Read the model definition and answer for the solid it produces. Units are mm, in the model's axes. A direction names the side the tool comes from. Coordinates: 2 decimals unless noted, no trailing zeros. Write each loop counter-clockwise with the first axis right and the second up, starting at its lowest first coordinate (ties: lowest second). Pieces come first, ordered by that corner, then holes. Notation, with made-up numbers: (51, 66) - (74, 66) arc R12 cw to (74, 74) - close; hole circle Ø10 at (40, -28.5). An arc over 180 degrees is marked (long way). Use a Markdown table: item, result.
Autodesk Inventor part; units mm, degrees
ref_plane "YZ Plane" through (0, 0, 0) normal (1, 0, 0) x (0, 1, 0)
ref_plane "XZ Plane" through (0, 0, 0) normal (0, 1, 0) x (-1, 0, 0)
ref_plane "XY Plane" through (0, 0, 0) normal (0, 0, 1) x (1, 0, 0)
sketch "Sketch1" plane through (0, 0, 0) normal (0, 1, 0) x (-1, 0, 0)
  line L0 (0, 0) -> (70, 0)
  line L1 (70, 0) -> (70, -10)
  line L2 (70, -10) -> (0, -10)
  line L3 (0, -10) -> (0, 0)
  line L4 (70, 0) -> (0, 0)
  line L5 (0, 0) -> (0, -5)
  line L6 (0, -5) -> (70, -5)
  line L7 (70, -5) -> (70, 0)
  line L8 (70, -5) -> (62, -5)
  line L9 (62, -5) -> (44, -5)
  line L10 (44, -5) -> (26, -5)
  line L11 (26, -5) -> (8, -5)
  line L12 (8, -5) -> (-6, -5)
  line L13 (70, 0) -> (90, 0)
  line L14 (90, 0) -> (90, -10)
  line L15 (90, -10) -> (70, -10)
  line L16 (70, -10) -> (70, 0)
  line L17 (0, -10) -> (-22, -10)
  line L18 (-22, -10) -> (-22, 0)
  line L19 (-22, 0) -> (0, 0)
  line L20 (0, 0) -> (0, -10)
  dimension "d0" = 70
  dimension "d1" = 10
  dimension "d2" = 5
  dimension "d3" = 8
  dimension "d4" = 18
  dimension "d5" = 18
  dimension "d6" = 18
  dimension "d22" = 20
  dimension "d23" = 22
extrude "Extrusion1" add sketch "Sketch1" along normal blind 40 contours L0 L1 L6 L3 | L6 L1 L2 L3
hole "Hole1" at (6, 0, -5) at (-8, 0, -5) at (-26, 0, -5) at (-44, 0, -5) at (-62, 0, -5) direction (0, 1, 0) diameter 3.242 depth 15 tip angle 118
extrude "Extrusion3" add sketch "Sketch1" along normal blind 86 contours L3 L17 L18 L19 | L13 L14 L15 L1
sketch "Sketch4" plane through (22, 0, -10) normal (0, 0, -1) x (-1, 0, 0)
  line L0 (112, 0) -> (112, 86)
  line L1 (112, 86) -> (101.5, 86)
  line L2 (101.5, 86) -> (101.5, 76)
  line L3 (101.5, 76) -> (112, 76)
  line L4 (112, 76) -> (112, 86)
  line L5 (0, 86) -> (22, 86)
  line L6 (0, 86) -> (8.5, 86)
  line L7 (8.5, 86) -> (8.5, 76)
  line L8 (8.5, 76) -> (0, 76)
  line L9 (0, 76) -> (0, 86)
  line L10 (22, 40) -> (92, 40)
  line L11 (22, 40) -> (55, 40)
  line L12 (55, 40) -> (55, 29.5)
  line L13 (55, 29.5) -> (22, 29.5)
  line L14 (22, 29.5) -> (22, 40)
  point P0 (22, 0)
  dimension "d35" = 10.5
  dimension "d36" = 10
  dimension "d44" = 8.5
  dimension "d45" = 10
  dimension "d46" = 10.5
  dimension "d47" = 33
hole "Hole3" at (-79.5, 76, -10) at (13.5, 76, -10) at (-33, 29.5, -10) direction (0, 0, 1) diameter 5.2 end through all counterbore diameter 10 counterbore depth 5
properties part number "CameraAdapter_part2"
(1) A cutting plane is placed at B-B, the plane y = 76. Write down the section's boundary in (x, z), and give its area (3 significant figures).
Report:
| item | result |
|---|---|
| outline | (-90, -10) - (-84.5, -10) - (-84.5, -5) - (-82.1, -5) - (-82.1, 0) - (-90, 0) - close; (-76.9, -5) - (-74.5, -5) - (-74.5, -10) - (-70, -10) - (-70, 0) - (-76.9, 0) - close; (0, -10) - (8.5, -10) - (8.5, -5) - (10.9, -5) - (10.9, 0) - (0, 0) - close; (16.1, -5) - (18.5, -5) - (18.5, -10) - (22, -10) - (22, 0) - (16.1, 0) - close |
| area | 268 mm² |
(2) For faces 4 (the flat face through (0, 63, -5)), 5 (the flat face through (-80, 86, -5)), 6 (the cylindrical face through (-45.607, 7.605, -4.789)), 7 (the cylindrical face through (-34.757, 27.584, -2.465)), 8 (the flat face through (16, 78, -5)), determine the directions among +Z, -Z, +X, -X, +Y, -Y from which every point of the face is accessible in a straight line to the end or side of a thin tool.
Report:
| item | result |
|---|---|
| face 4 | +Z, -Z, +Y |
| face 5 | +Z, -Z, +X, -X, +Y |
| face 6 | -Y |
| face 7 | +Z, -Z |
| face 8 | -Z |
(3) A cutting plane is placed at D-D, the plane y = 28.5. Write down the section's boundary in (x, z).
Report:
| item | result |
|---|---|
| outline | (-90, -10) - (-37.9, -10) - (-37.9, -5) - (-35.4, -5) - (-35.4, 0) - (-90, 0) - close; (-30.6, -5) - (-28.1, -5) - (-28.1, -10) - (22, -10) - (22, 0) - (-30.6, 0) - close |
(4) Each of these flat-tipped pins is pushed along its axis until it touches: P1, Ø5, axis at x = -26, z = -5, coming from the +Y side; P2, Ø4, axis at x = -33, y = 29.5, coming from the +Z side; P3, Ø6, axis at x = -79.5, y = 76, coming from the -Z side. Where does it stop, or does it pass through?
Report:
| item | result |
|---|---|
| P1 | stops at y = 40 |
| P2 | passes through |
| P3 | stops at z = -5 |
(5) A cutting plane is placed at C-C, the plane z = -1.75. Write down the section's boundary in (x, y).
Report:
| item | result |
|---|---|
| outline | (-90, 0) - (22, 0) - (22, 86) - (0, 86) - (0, 40) - (-70, 40) - (-70, 86) - (-90, 86) - close; hole circle Ø5.2 at (-79.5, 76); hole circle Ø5.2 at (-33, 29.5); hole circle Ø5.2 at (13.5, 76) |
(6) Straight lines are drawn through the part: L1, parallel to X at y = 76, z = -8.4; L2, parallel to X at y = 76, z = -1.8; L3, parallel to X at y = 6.75, z = -5. For each, find the intervals that lie inside material, in ascending order.
Report:
| item | result |
|---|---|
| L1 | x = -90 to -84.5, -74.5 to -70, 0 to 8.5, 18.5 to 22 |
| L2 | x = -90 to -82.1, -76.9 to -70, 0 to 10.9, 16.1 to 22 |
| L3 | x = -90 to -63.62, -60.38 to -45.62, -42.38 to -27.62, -24.38 to -9.62, -6.38 to 22 |
(7) A cutting plane is placed at A-A, the plane x = 13.5. Write down the section's boundary in (y, z), and give its area (3 significant figures).
Report:
| item | result |
|---|---|
| outline | (0, -10) - (71, -10) - (71, -5) - (73.4, -5) - (73.4, 0) - (0, 0) - close; (78.6, -5) - (81, -5) - (81, -10) - (86, -10) - (86, 0) - (78.6, 0) - close |
| area | 784 mm² |
(8) The mould has two halves that part along X. Classify faces 1 (the flat face through (-33, 33, 0)), 2 (the flat face through (-90, 42, -5)), 3 (the cylindrical face through (-60.418, 7.605, -4.649)): pulls with the +X half, pulls with the -X half, needs draft (parallel to the pull), parting line crosses it, or undercut.
Report:
| item | result |
|---|---|
| face 1 | needs draft |
| face 2 | pulls with the -X half |
| face 3 | undercut |
